Autodesk Inventor part; units mm, degrees
ref_plane "YZ Plane" through (0, 0, 0) normal (1, 0, 0) x (0, 1, 0)
ref_plane "XZ Plane" through (0, 0, 0) normal (0, 1, 0) x (-1, 0, 0)
ref_plane "XY Plane" through (0, 0, 0) normal (0, 0, 1) x (1, 0, 0)
sketch "Esquisse1" plane through (0, 0, 0) normal (0, 1, 0) x (-1, 0, 0)
  circle A0 centre (0, 0) radius 25 construction
  line L0 (-25, 0) -> (25, 0) construction
  arc A1 (-75, -80.7775) -> (-75, 80.7775) centre (-25, 0) ccw construction
  arc A2 (75, 80.7775) -> (75, -80.7775) centre (25, 0) ccw construction
  line L1 (0, 25) -> (0, 0) construction
  line L2 (-75, 80.7775) -> (75, 80.7775)
  line L3 (-75, -80.7775) -> (75, -80.7775)
  arc A3 (75, -80.7775) -> (75, 80.7775) centre (25, 0) ccw
  arc A4 (-75, 80.7775) -> (-75, -80.7775) centre (-25, 0) ccw
  dimension "d0" = 50
  dimension "d1" = 190
  dimension "d2" = 150
extrude "Extrusion1" add sketch "Esquisse1" along normal blind 4
sketch "Esquisse2" plane through (0, 4, 0) normal (0, 1, 0) x (1, 0, 0)
  line L0 (75, 80.7775) -> (-75, 80.7775)
  arc A0 (-75, 80.7775) -> (-75, -80.7775) centre (-25, 0) ccw
  line L1 (-95, 32.5) -> (-60, 32.5)
  line L2 (-60, 32.5) -> (-60, -32.5)
  line L3 (-60, -32.5) -> (-95, -32.5)
  line L4 (-95, -32.5) -> (-95, 32.5)
  line L5 (60, 32.5) -> (95, 32.5)
  line L6 (95, 32.5) -> (95, -32.5)
  line L7 (95, -32.5) -> (60, -32.5)
  line L8 (60, -32.5) -> (60, 32.5)
  line L9 (0, 0) -> (0, 80.7775) construction
  line L10 (0, 0) -> (-120, 0) construction
  dimension "d5" = 35
  dimension "d6" = 60
  dimension "d7" = 65
extrude "Extrusion2" cut sketch "Esquisse2" against normal through all
sketch "Esquisse3" plane through (0, 4, 0) normal (0, 1, 0) x (1, 0, 0)
  line L0 (75, 80.7775) -> (-75, 80.7775)
  circle A0 centre (-88, 45) radius 3
  circle A1 centre (-88, -45) radius 3
  line L1 (-88, -45) -> (-88, 45) construction
  line L2 (0, 0) -> (-88, 0) construction
  line L3 (0, 0) -> (0, 80.7775) construction
  circle A2 centre (88, 45) radius 3
  circle A3 centre (88, -45) radius 3
  dimension "d10" = 88
  dimension "d11" = 6
  dimension "d12" = 90
extrude "Extrusion3" cut sketch "Esquisse3" against normal through all
sketch "Esquisse4" plane through (0, 0, 0) normal (0, -1, 0) x (1, 0, 0)
  line L0 (-50, 50) -> (50, 50) construction
  line L1 (50, 50) -> (50, -50) construction
  line L2 (50, -50) -> (-50, -50) construction
  line L3 (-50, -50) -> (-50, 50) construction
  circle A0 centre (-50, 50) radius 3
  circle A1 centre (50, 50) radius 3
  circle A2 centre (50, -50) radius 3
  circle A3 centre (-50, -50) radius 3
  line L4 (75, 80.7775) -> (-75, 80.7775)
  point P0 (0, 0)
  dimension "d15" = 100
  dimension "d16" = 100
  dimension "d17" = 50
  dimension "d18" = 50
  dimension "d19" = 6
  dimension "d20" = 6
  dimension "d21" = 6
  dimension "d22" = 6
  dimension "d25" = 30.7775
extrude "Extrusion4" cut sketch "Esquisse4" against normal through all
equation "\"d20\" = d19"
equation "\"d21\" = d19"
equation "\"d22\" = d19"
properties part number "base"
Input: part model. Units: mm. Frame: model coordinates. Coordinates: 2 decimals unless noted, no trailing zeros. Order: outer loops, then holes, each group sorted by start corner. A loop starts at its lowest first (then second) coordinate and runs counter-clockwise, first axis right, second up.
1. Cut plane C-C, the plane x = 50. Return loops of the section in (y, z).
Checked values:
outline: (0, -80.78) - (4, -80.78) - (4, -53) - (0, -53) - close; (0, -47) - (4, -47) - (4, 47) - (0, 47) - close; (0, 53) - (4, 53) - (4, 80.78) - (0, 80.78) - close
2. Ray query, line 1 along Z through (x, y) = (74.5, 3.3); line 2 along X through (y, z) = (2.8, 10.5); line 3 along Z through (x, y) = (88, 2.8). Return the intervals inside material, ascending.
Checked values:
line 1: z = -80.78 to -32.5, 32.5 to 80.78
line 2: x = -119.42 to -95, -60 to 60, 95 to 119.42
line 3: z = -71.11 to -48, -42 to -32.5, 32.5 to 42, 48 to 71.11
3. Draft query along X for faces 1 (the cylindrical face through (-119.99, 1.97, 1.35)), 2 (the flat face through (2, 4, 1)), 3 (the cylindrical face through (-91, 2, 45)). Return one class per face: +X half, -X half, draft (parallel to the pull), parting line (faces both ways), or undercut.
Checked values:
face 1: -X half
face 2: draft
face 3: undercut
4. Cut plane B-B, the plane z = 0.5. Return loops of the section in (x, y).
Checked values:
outline: (-120, 0) - (-95, 0) - (-95, 4) - (-120, 4) - close; (-60, 0) - (60, 0) - (60, 4) - (-60, 4) - close; (95, 0) - (120, 0) - (120, 4) - (95, 4) - close
5. Cut plane D-D, the plane x = 77.5. Return loops of the section in (y, z), plus the area to 3 significant figures.
Checked values:
outline: (0, -79.18) - (4, -79.18) - (4, -32.5) - (0, -32.5) - close; (0, 32.5) - (4, 32.5) - (4, 79.18) - (0, 79.18) - close
area: 373 mm2
6. Cut plane A-A, the plane y = 0.8. Count the separate pieces of the cut face and the enclosed holes in it, plus the area to 3 significant figures.
Checked values:
separate pieces: 1
enclosed holes: 10
area: 29,700 mm2
7. Contact query for flat-ended pins moving along their axis: P1, Ø2, axis at y = 1.5, z = 33.5, coming from the -X side; P2, Ø2, axis at x = 77, y = 1.5, coming from the +Z side; P3, Ø2, axis at y = 2.5, z = 3.5, coming from the +X side. Output: stop coordinate, or through.
Checked values:
P1: stops at x = -114.27
P2: stops at z = 80.15
P3: stops at x = 119.97
